Work out the finished part from the listing and answer in its coordinate system (mm). A direction names the side the tool comes from. Give positions to 0.01 mm unless a question says otherwise; leave off trailing zeros. Write each loop counter-clockwise with the first axis right and the second up, starting at its lowest first coordinate (ties: lowest second). Pieces come first, ordered by that corner, then holes.
1) Find section C-C (y = 4). Determine the outline of the cut face in (x, z).
2) Find section D-D (x = 19). Determine the outline of the cut face in (y, z), plus the area to 3 significant figures.
3) Determine the mould class of faces 1 (the face through (16.834, 19.243, 1.517)), 2 (the face through (-21.302, 9.164, 5.063)), 3 (the face through (-27, 9, 8)) for opening direction Z: pulls with the +Z half, pulls with the -Z half, needs draft (parallel to the pull), parting line crosses it, or undercut.
4) Given pin 1 Ø7 at (x, z) = (13.5, -7) entering from +Y; pin 2 Ø0.8 at (x, y) = (23, 11) entering from -Z; pin 3 Ø2.5 at (x, z) = (10, 0) entering from -Y, each flat-ended and moving along its own axis, determine where each tip first touches the part or whether it passes through.
5) Find section B-B (x = -24.3). Determine the outline of the cut face in (y, z).
6) A tool of negligible diameter and unlimited length cuts with its end or side. For faces 4 (the face through (-21, 10.15, 5)), 5 (the face through (18, 16.75, -8)), 6 (the face through (-20, -4, 0)), 7 (the face through (12.44, 22.57, 0.54)), from which of +Z, -Z, +X, -X, +Y, -Y can it reach the whole face along a straight path? Write none if from no direction.
7) Find section A-A (x = 10). Determine the outline of the cut face in (y, z), plus the area to 3 significant figures.
8) Straight lines are drawn through the part: probe 1 along Z at (x, y) = (-24, 9); probe 2 along Y at (x, z) = (4, -4.25); probe 3 along X at (y, z) = (5, -6.25). For each, find the intervals that lie inside material, in ascending order.
```python
from build123d import *

# Parameters (mm, degrees)
SKETCH_2_W          = 40
SKETCH_2_H          = 37.5
EXTRUDE_1_DEPTH     = 9.95
SKETCH_3_W          = 7
SKETCH_3_H          = 2
EXTRUDE_2_DEPTH     = 19.9
EXTRUDE_2_2_DEPTH   = 19.9
SKETCH_4_R          = 3
CUT_EXTRUDE_1_DEPTH = 19.9
SKETCH_5_W          = 7
SKETCH_5_H          = 1
EXTRUDE_3_DEPTH     = 1
CUT_EXTRUDE_2_DEPTH = 35.492970298
CUT_EXTRUDE_6_DEPTH = 2
CUT_EXTRUDE_7_DEPTH = 2
SKETCH_10_R         = 2.5
SKETCH_10_R_2       = 2
EXTRUDE_4_DEPTH     = 6.2
SKETCH_11_R         = 7
EXTRUDE_5_DEPTH     = 1
SKETCH_12_R         = 5
EXTRUDE_6_DEPTH     = 0.5
EXTRUDE_START       = 6.2
SKETCH_13_R         = 2.5
SKETCH_13_R_2       = 2
EXTRUDE_7_DEPTH     = 6.2
CHAMFER_1_SIZE      = 2


with BuildPart() as part:
    # Sketch 2 → Extrude 1 (new, symmetric)
    with BuildSketch(Plane.XY):
        Rectangle(SKETCH_2_W, SKETCH_2_H)
    extrude(amount=EXTRUDE_1_DEPTH, both=True)



with BuildPart() as body_2:
    # Sketch 3 → Extrude 2 (new body)
    with BuildSketch(Plane.XY.offset(9.95)):
        with Locations((23.5, 9.15)):
            Rectangle(SKETCH_3_W, SKETCH_3_H)
    extrude(amount=-EXTRUDE_2_DEPTH)


with BuildPart() as body_3:
    # Sketch 3 → Extrude 2 2 (new body)
    with BuildSketch(Plane.XY.offset(9.95)):
        with Locations((-23.5, 9.15)):
            Rectangle(SKETCH_3_W, SKETCH_3_H)
    extrude(amount=-EXTRUDE_2_2_DEPTH)


with BuildPart() as cut_extrude_1_tool:
    # Sketch 4 → Cut-Extrude 1 (new body)
    with BuildSketch(Plane(origin=(0, 10.15, 0), x_dir=(1, 0, 0), z_dir=(0, 1, 0))):
        with Locations((-24.3, 4.95)):
            Circle(SKETCH_4_R)
        with Locations((24.3, 4.95)):
            Circle(SKETCH_4_R)
        with Locations((24.3, -4.95)):
            Circle(SKETCH_4_R)
        with Locations((-24.3, -4.95)):
            Circle(SKETCH_4_R)
    extrude(amount=-CUT_EXTRUDE_1_DEPTH)


with BuildPart() as body_2_1:
    add(body_2.part)

    # Cut-Extrude 1: cut by cut_extrude_1_tool
    add(cut_extrude_1_tool.part, mode=Mode.SUBTRACT)


with BuildPart() as body_3_1:
    add(body_3.part)

    # Cut-Extrude 1: cut by cut_extrude_1_tool
    add(cut_extrude_1_tool.part, mode=Mode.SUBTRACT)


with BuildPart() as part_1:
    add(part.part)

    add(body_2_1.part)  # Extrude 3 merges body 2

    add(body_3_1.part)  # Extrude 3 merges body 3
    # Sketch 5 → Extrude 3 (add)
    with BuildSketch(Plane(origin=(0, 10.15, 0), x_dir=(1, 0, 0), z_dir=(0, 1, 0))):
        Polygon((-27, 0), (-27, 0.5), (-20, 0.5), (-20, -0.5), (-27, -0.5), align=None)
        with Locations((23.5, 0)):
            Rectangle(SKETCH_5_W, SKETCH_5_H)
    extrude(amount=EXTRUDE_3_DEPTH)

    # Sketch 6 → Cut-Extrude 2 (cut, through all)
    with BuildSketch(Plane.XY.offset(0.5)):
        Polygon((20, 11.15), (27, 10.15), (27, 11.15), align=None)
        Polygon((-27, 10.15), (-27, 11.15), (-20, 11.15), align=None)
    extrude(amount=-CUT_EXTRUDE_2_DEPTH, mode=Mode.SUBTRACT)

    # Sketch 8 → Cut-Extrude 6 (cut)
    with BuildSketch(Plane(origin=(0, 18.75, 0), x_dir=(1, 0, 0), z_dir=(0, 1, 0))):
        Polygon((-20, 9.95), (-20, -9.95), (-14, -9.95), (-14, -9.85), (-14, 9.85), (-14, 9.95), align=None)
    extrude(amount=-CUT_EXTRUDE_6_DEPTH, mode=Mode.SUBTRACT)

    # Sketch 9 → Cut-Extrude 7 (cut)
    with BuildSketch(Plane(origin=(0, 18.75, 0), x_dir=(1, 0, 0), z_dir=(0, 1, 0))):
        with BuildLine():
            Line((20, 1.9e-08), (20, 9.95))
            Line((20, 9.95), (10.998749218, 9.95))
            ThreePointArc((10.998749218, 9.95), (17.41577683, 6.708670062), (20, 1.9e-08))
        make_face()
        with BuildLine():
            Line((20, -9.95), (20, 1.9e-08))
            ThreePointArc((20, 1.9e-08), (17.415776843, -6.708670048), (10.998749218, -9.95))
            Line((10.998749218, -9.95), (20, -9.95))
        make_face()
    extrude(amount=-CUT_EXTRUDE_7_DEPTH, mode=Mode.SUBTRACT)

    # Sketch 10 → Extrude 4 (add)
    with BuildSketch(Plane(origin=(0, 18.75, 0), x_dir=(1, 0, 0), z_dir=(0, 1, 0))):
        with Locations(Location((10, 0, 0), (0, 0, 90))):
            Circle(SKETCH_10_R)
        with Locations(Location((10, 0, 0), (0, 0, 90))):
            Circle(SKETCH_10_R_2, mode=Mode.SUBTRACT)
    extrude(amount=EXTRUDE_4_DEPTH)

    # Sketch 11 → Extrude 5 (add)
    with BuildSketch(Plane(origin=(0, 18.75, 0), x_dir=(1, 0, 0), z_dir=(0, 1, 0))):
        with Locations(Location((10, 0, 0), (0, 0, 90))):
            Circle(SKETCH_11_R)
    extrude(amount=EXTRUDE_5_DEPTH)

    # Sketch 12 → Extrude 6 (add)
    with BuildSketch(Plane(origin=(0, 19.75, 0), x_dir=(1, 0, 0), z_dir=(0, 1, 0))):
        with Locations(Location((10, 0, 0), (0, 0, 270))):
            Circle(SKETCH_12_R)
    extrude(amount=EXTRUDE_6_DEPTH)

    # Sketch 13 → Extrude 7 (add)
    with BuildSketch(Plane.XZ.offset(18.75).offset(EXTRUDE_START)):
        with Locations(Location((10, 0, 0), (0, 0, 270))):
            Circle(SKETCH_13_R)
        with Locations(Location((10, 0, 0), (0, 0, 270))):
            Circle(SKETCH_13_R_2, mode=Mode.SUBTRACT)
    extrude(amount=-EXTRUDE_7_DEPTH)

    # Chamfer 1
    chamfer_1_edges = [part_1.edges().sort_by_distance(p)[0] for p in [
        (20, -18.75, 0),
        (-20, -18.75, 0),
    ]]
    chamfer(chamfer_1_edges, length=CHAMFER_1_SIZE)


solid = part_1.part
```
Results:
1. outline: (-20, -9.95) - (20, -9.95) - (20, 9.95) - (-20, 9.95) - close
2. outline: (-17.75, -9.95) - (16.75, -9.95) - (16.75, -4.36) - (18.75, -4.36) - (18.75, 4.36) - (16.75, 4.36) - (16.75, 9.95) - (-17.75, 9.95) - close
2. area: 704 mm2
3. face 1: parting line crosses it
3. face 2: undercut
3. face 3: needs draft
4. pin 1: stops at y = 20.25
4. pin 2: stops at z = -0.5
4. pin 3: stops at y = -18.75
5. outline: (8.15, -9.95) - (10.15, -9.95) - (10.15, -7.95) - (8.15, -7.95) - close; (8.15, -1.95) - (10.15, -1.95) - (10.15, -0.5) - (10.54, -0.5) - (10.54, 0.5) - (10.15, 0.5) - (10.15, 1.95) - (8.15, 1.95) - close; (8.15, 7.95) - (10.15, 7.95) - (10.15, 9.95) - (8.15, 9.95) - close
6. face 4: +Z, -X, +Y
6. face 5: -Z, +X, +Y
6. face 6: +Z, -Z, -X, -Y
6. face 7: +Y
7. outline: (-24.95, -2.5) - (-18.75, -2.5) - (-18.75, -9.95) - (18.75, -9.95) - (18.75, -7) - (19.75, -7) - (19.75, -5) - (20.25, -5) - (20.25, -2.5) - (24.95, -2.5) - (24.95, -2) - (20.25, -2) - (20.25, 2) - (24.95, 2) - (24.95, 2.5) - (20.25, 2.5) - (20.25, 5) - (19.75, 5) - (19.75, 7) - (18.75, 7) - (18.75, 9.95) - (-18.75, 9.95) - (-18.75, 2.5) - (-24.95, 2.5) - (-24.95, 2) - (-18.75, 2) - (-18.75, -2) - (-24.95, -2) - close
7. area: 776 mm2
8. probe 1: z = -9.95 to -7.93, -1.97 to 1.97, 7.93 to 9.95
8. probe 2: y = -18.75 to 18.75
8. probe 3: x = -20 to 20
